```python
from build123d import *

# Parameters (mm, degrees)
SKETCH_1_R                = 19
EXTRUDE_1_DEPTH           = 40
CUT_EXTRUDE_1_DEPTH       = 49.187135213
CUT_EXTRUDE_1_DEPTH_BACK  = 49.187135213
SKETCH_2_OUTSIDE_W        = 55.398
SKETCH_2_OUTSIDE_H        = 53.398
SKETCH_3_R                = 1.75
CUT_EXTRUDE_2_DEPTH       = 7.4
CUT_EXTRUDE_4_DEPTH       = 5
SKETCH_6_W                = 6.3
SKETCH_6_H                = 6.3
CUT_EXTRUDE_5_DEPTH       = 1.2
SKETCH_10_R               = 1.4
CUT_EXTRUDE_8_DEPTH       = 13.7
CUT_EXTRUDE_9_REACH       = 35.156
SKETCH_11_R               = 0.8
SKETCH_12_W               = 8
SKETCH_12_H               = 2.5
CUT_EXTRUDE_10_DEPTH      = 27.566913633
SKETCH_13_R               = 0.5
CUT_EXTRUDE_11_DEPTH      = 1.2
CUT_EXTRUDE_12_DEPTH      = 27.566913633
CUT_EXTRUDE_12_DEPTH_BACK = 27.566913633
SKETCH_14_W               = 31.188232258
SKETCH_14_H               = 3.19353307


with BuildPart() as part:
    # 草图1 → 凸台-拉伸1 (new body)
    with BuildSketch(Plane(origin=(0, 0, 0), x_dir=(0, 0, -1), z_dir=(1, 0, 0))):
        Circle(SKETCH_1_R)
    extrude(amount=EXTRUDE_1_DEPTH)

    # 草图2 outside → 切除-拉伸1 (cut, two sides: drawn at the far end of the back side and taken through both)
    with BuildSketch(Plane.XY.offset(-CUT_EXTRUDE_1_DEPTH_BACK)):
        with Locations((20, 0)):
            Rectangle(SKETCH_2_OUTSIDE_W, SKETCH_2_OUTSIDE_H)
        Polygon((12.186055083, 1.5), (14.466055083, 1.5), (23.466055083, 1.5), (23.466055083, -7.5), (23.466055083, -14.75), (12.186055083, -14.75), align=None, mode=Mode.SUBTRACT)
    extrude(amount=CUT_EXTRUDE_1_DEPTH + CUT_EXTRUDE_1_DEPTH_BACK, mode=Mode.SUBTRACT)

    # 草图3 → 切除-拉伸2 (cut)
    with BuildSketch(Plane.ZY.offset(-12.186055083)):
        with Locations((0, -3)):
            Circle(SKETCH_3_R)
    extrude(amount=-CUT_EXTRUDE_2_DEPTH, mode=Mode.SUBTRACT)

    # 草图5 → 切除-拉伸4 (cut, symmetric)
    with BuildSketch(Plane.XY):
        Polygon((14.466055083, 1.5), (23.466055083, -7.5), (23.466055083, 1.5), align=None)
    extrude(amount=CUT_EXTRUDE_4_DEPTH, both=True, mode=Mode.SUBTRACT)

    # 草图6 → 切除-拉伸5 (cut)
    with BuildSketch(Plane(origin=(7.983027542, 7.983027542, 0), x_dir=(0, 0, -1), z_dir=(0.7071067811865487, 0.7071067811865465, 0))):
        with Locations((0, -14.958385475)):
            Rectangle(SKETCH_6_W, SKETCH_6_H)
    extrude(amount=-CUT_EXTRUDE_5_DEPTH, mode=Mode.SUBTRACT)

    # 草图10 → 切除-拉伸8 (cut)
    with BuildSketch(Plane.XZ.offset(14.75)):
        with Locations((13.686055083, 10.5)):
            Circle(SKETCH_10_R)
        with Locations((21.966055083, 10.5)):
            Circle(SKETCH_10_R)
        with Locations((13.686055083, -10.5)):
            Circle(SKETCH_10_R)
        with Locations((21.966055083, -10.5)):
            Circle(SKETCH_10_R)
    extrude(amount=-CUT_EXTRUDE_8_DEPTH, mode=Mode.SUBTRACT)

    # 草图11 → 切除-拉伸9 (cut, up to next)
    with BuildSketch(Plane.XZ.offset(1.05), mode=Mode.PRIVATE) as cut_extrude_9_sk1:
        with Locations((13.686055083, 10.5)):
            Circle(SKETCH_11_R)
    cut_extrude_9_tool1 = extrude(cut_extrude_9_sk1.sketch, amount=-CUT_EXTRUDE_9_REACH, mode=Mode.PRIVATE) & part.part
    # 草图11 → 切除-拉伸9 (cut, up to next)
    with BuildSketch(Plane.XZ.offset(1.05), mode=Mode.PRIVATE) as cut_extrude_9_sk2:
        with Locations((21.966055083, 10.5)):
            Circle(SKETCH_11_R)
    cut_extrude_9_tool2 = extrude(cut_extrude_9_sk2.sketch, amount=-CUT_EXTRUDE_9_REACH, mode=Mode.PRIVATE) & part.part
    # 草图11 → 切除-拉伸9 (cut, up to next)
    with BuildSketch(Plane.XZ.offset(1.05), mode=Mode.PRIVATE) as cut_extrude_9_sk3:
        with Locations((13.686055083, -10.5)):
            Circle(SKETCH_11_R)
    cut_extrude_9_tool3 = extrude(cut_extrude_9_sk3.sketch, amount=-CUT_EXTRUDE_9_REACH, mode=Mode.PRIVATE) & part.part
    # 草图11 → 切除-拉伸9 (cut, up to next)
    with BuildSketch(Plane.XZ.offset(1.05), mode=Mode.PRIVATE) as cut_extrude_9_sk4:
        with Locations((21.966055083, -10.5)):
            Circle(SKETCH_11_R)
    cut_extrude_9_tool4 = extrude(cut_extrude_9_sk4.sketch, amount=-CUT_EXTRUDE_9_REACH, mode=Mode.PRIVATE) & part.part
    add(cut_extrude_9_tool1.solids().sort_by_distance((13.686055, -1.05, 10.5))[0], mode=Mode.SUBTRACT)
    add(cut_extrude_9_tool2.solids().sort_by_distance((21.966055, -1.05, 10.5))[0], mode=Mode.SUBTRACT)
    add(cut_extrude_9_tool3.solids().sort_by_distance((13.686055, -1.05, -10.5))[0], mode=Mode.SUBTRACT)
    add(cut_extrude_9_tool4.solids().sort_by_distance((21.966055, -1.05, -10.5))[0], mode=Mode.SUBTRACT)

    # 草图12 → 切除-拉伸10 (cut, through all)
    with BuildSketch(Plane(origin=(23.466055083, 0, 0), x_dir=(0, 0, -1), z_dir=(1, 0, 0))):
        with Locations((0, -13.5)):
            Rectangle(SKETCH_12_W, SKETCH_12_H)
    extrude(amount=-CUT_EXTRUDE_10_DEPTH, mode=Mode.SUBTRACT)

    # 草图13 → 切除-拉伸11 (cut)
    with BuildSketch(Plane(origin=(7.983027542, 7.983027542, 0), x_dir=(0, 0, -1), z_dir=(0.7071067811865487, 0.7071067811865465, 0))):
        with Locations((-3.15, -11.808385475)):
            Circle(SKETCH_13_R)
        with Locations((3.15, -11.808385475)):
            Circle(SKETCH_13_R)
        with Locations((-3.15, -18.108385475)):
            Circle(SKETCH_13_R)
        with Locations((3.15, -18.108385475)):
            Circle(SKETCH_13_R)
    extrude(amount=-CUT_EXTRUDE_11_DEPTH, mode=Mode.SUBTRACT)

    # 草图14 → 切除-拉伸12 (cut, two sides: drawn at the far end of the back side and taken through both)
    with BuildSketch(Plane.ZY.offset(-12.186055083).offset(-CUT_EXTRUDE_12_DEPTH_BACK)):
        with Locations((-0.125755843, -14.846766535)):
            Rectangle(SKETCH_14_W, SKETCH_14_H)
    extrude(amount=CUT_EXTRUDE_12_DEPTH + CUT_EXTRUDE_12_DEPTH_BACK, mode=Mode.SUBTRACT)


solid = part.part
```
The model under review builds one solid part; all positions refer to its coordinate system, in mm. A direction names the side the tool comes from. Coordinates: 2 decimals unless noted, no trailing zeros. Write each loop counter-clockwise with the first axis right and the second up, starting at its lowest first coordinate (ties: lowest second). Pieces come first, ordered by that corner, then holes. Notation, with made-up numbers: (69.25, 69) -> (121.25, 69) arc R30 cw to (121.25, 100) -> close; hole circle Ø5 at (3, 43.5). An arc over 180 degrees is marked (long way). One line per item, written item: value. Start each with the question number.
Q1. The part is to be moulded in two halves that separate along Y. For faces 1 (the face through (20.37, -5.24, 0.04)), 2 (the face through (21, -1, 5)), 3 (the face through (20.63, -5.5, -3.49)), say which applies: +Y half, -Y half, draft (parallel to the pull), parting line (faces both ways), or undercut.
Q2. To check wall thickness, follow probe 1 along X at (y, z) = (-4, 10); probe 2 along Z at (x, y) = (22, -8.5); probe 3 along Z at (x, y) = (13.5, -0.75). State the ranges of each line that lie inside material, in increasing order.
Q3. For faces 4 (the face through (14.44, -7.24, 11.68)), 5 (the face through (18, -13, -4)), 6 (the face through (15.9, -0.8, 0)), list the 3-axis set-ups (+Z, -Z, +X, -X, +Y, -Y) from which the entire face can be reached by the end or side of a thin tool; tool diameter is ignored.
Q4. Add section B-B, the plane z = 10.5. Give the boundary of the cut face in (x, y), then the cut area to 3 significant figures.
Q5. Clearance check with flat-ended pins moving along their axes: P1, Ø1.4, axis at x = 14, z = -10, coming from the -Y side; P2, Ø3, axis at x = 15, y = -10.5, coming from the +Z side; P3, Ø1.4, axis at x = 17.5, y = -2, coming from the -Z side. State where each tip first meets the part, or that it passes through.
Q6. Add section A-A, the plane y = -4. Give the boundary of the cut face in (x, z).
Q7. Add section D-D, the plane y = -9.75. Give the boundary of the cut face in (x, z).
Q8. Add section C-C, the plane z = 0. Give the boundary of the cut face in (x, y), then the cut area to 3 significant figures.
Response:
1. face 1: +Y half
1. face 2: draft
1. face 3: undercut
2. probe 1: 12.19 to 12.38, 14.99 to 20.66, 23.27 to 23.47
2. probe 2: -16.99 to -11.9, -9.1 to 9.1, 11.9 to 16.99
2. probe 3: -18.99 to -11.28, -9.72 to 9.72, 11.28 to 18.99
3. face 4: -Y
3. face 5: +X, -X, -Y
3. face 6: +X
4. outline: (12.19, -13.25) -> (12.29, -13.25) -> (12.29, -1.05) -> (12.89, -1.05) -> (12.89, 1.5) -> (12.19, 1.5) -> close; (14.49, -1.05) -> (15.09, -1.05) -> (15.09, -13.25) -> (20.57, -13.25) -> (20.57, -1.05) -> (21.17, -1.05) -> (21.17, 1.5) -> (14.49, 1.5) -> close; (22.77, -1.05) -> (23.37, -1.05) -> (23.37, -13.25) -> (23.47, -13.25) -> (23.47, 1.5) -> (22.77, 1.5) -> close
4. area: 89.9 mm²
5. P1: y = -1.05
5. P2: z = 16.73
5. P3: z = -18.96
6. outline: (12.19, -18.57) -> (23.47, -18.57) -> (23.47, -5) -> (19.97, -5) -> (19.97, -3.15) -> (18.27, -3.15) -> (18.27, -1.44) -> (12.19, -1.44) -> close; (12.19, 1.44) -> (18.27, 1.44) -> (18.27, 3.15) -> (19.97, 3.15) -> (19.97, 5) -> (23.47, 5) -> (23.47, 18.57) -> (12.19, 18.57) -> close; hole circle Ø2.8 at (13.69, -10.5); hole circle Ø2.8 at (13.69, 10.5); hole circle Ø2.8 at (21.97, -10.5); hole circle Ø2.8 at (21.97, 10.5)
7. outline: (12.19, -16.31) -> (23.47, -16.31) -> (23.47, 16.31) -> (12.19, 16.31) -> close; hole circle Ø2.8 at (13.69, -10.5); hole circle Ø2.8 at (13.69, 10.5); hole circle Ø2.8 at (21.97, -10.5); hole circle Ø2.8 at (21.97, 10.5)
8. outline: (12.19, -12.25) -> (23.47, -12.25) -> (23.47, -7.5) -> (20.79, -4.82) -> (19.94, -5.67) -> (19.02, -4.75) -> (12.19, -4.75) -> close; (12.19, -1.25) -> (15.52, -1.25) -> (15.48, -1.22) -> (16.33, -0.37) -> (14.47, 1.5) -> (12.19, 1.5) -> close
8. area: 89.2 mm²
